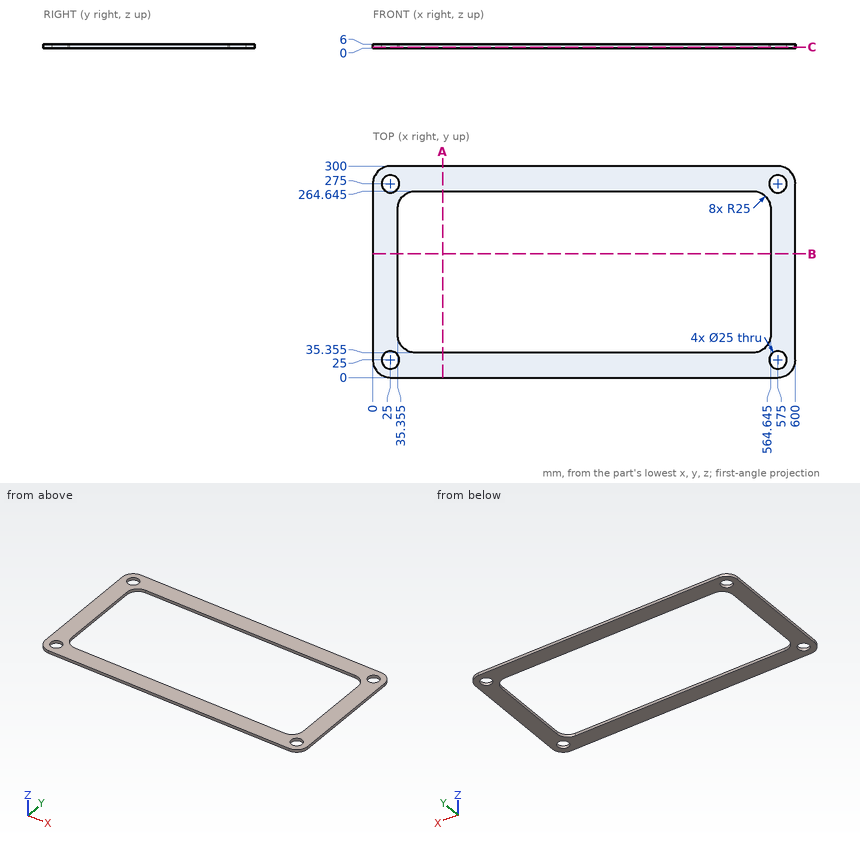
Geometry: see drawing. Coordinates: mm, zero at the bounding-box minimum. Coordinates: 2 decimals unless noted, no trailing zeros. Loops run counter-clockwise (first coordinate to the right, second up) from the corner with the lowest first, then second, coordinate; pieces in that order, holes last. Notation, with made-up numbers: (56, 38) - (74, 38) arc R11 cw to (74, 46) - close; hole circle Ø5 at (-23, 23.5). An arc over 180 degrees is marked (long way). Return JSON: item names as keys, results as strings.
Q1. Section A-A, the plane x = 99. Return loops of the section in (y, z) (1 decimal).
Results:
{"outline": "(0, 0) - (35.4, 0) - (35.4, 6) - (0, 6) - close; (264.6, 0) - (300, 0) - (300, 6) - (264.6, 6) - close"}
Q2. Section B-B, the plane y = 175.5. Return loops of the section in (x, z) (1 decimal).
Results:
{"outline": "(0, 0) - (35.4, 0) - (35.4, 6) - (0, 6) - close; (564.6, 0) - (600, 0) - (600, 6) - (564.6, 6) - close"}
Q3. Material intervals for line 1 along X through (y, z) = (275, 4.25); line 2 along Y through (x, z) = (575, 4.4); line 3 along Y through (x, z) = (506.5, 4.65) (1 decimal), sorted ascending.
Results:
{"line 1": "0 to 12.5, 37.5 to 562.5, 587.5 to 600", "line 2": "0 to 12.5, 37.5 to 262.5, 287.5 to 300", "line 3": "0 to 35.4, 264.6 to 300"}
Q4. Section C-C, the plane z = 1.5. Return loops of the section in (x, y) (1 decimal).
Results:
{"outline": "(0, 25) arc R25 ccw to (25, 0) - (575, 0) arc R25 ccw to (600, 25) - (600, 275) arc R25 ccw to (575, 300) - (25, 300) arc R25 ccw to (0, 275) - close; hole circle Ø25 at (25, 25); hole circle Ø25 at (25, 275); hole (35.4, 60.4) arc R25 ccw to (60.4, 35.4) - (539.6, 35.4) arc R25 ccw to (564.6, 60.4) - (564.6, 239.6) arc R25 ccw to (539.6, 264.6) - (60.4, 264.6) arc R25 ccw to (35.4, 239.6) - close; hole circle Ø25 at (575, 25); hole circle Ø25 at (575, 275)"}
